Work out the finished part from the listing and answer in its coordinate system (mm). A direction names the side the tool comes from. Coordinates: 2 decimals unless noted, no trailing zeros. Write each loop counter-clockwise with the first axis right and the second up, starting at its lowest first coordinate (ties: lowest second). Pieces come first, ordered by that corner, then holes. Notation, with made-up numbers: (63.25, 73.25) - (112.25, 73.25) arc R9 ccw to (112.25, 83.25) - close; hole circle Ø1 at (74, -34). An arc over 180 degrees is marked (long way). Use a Markdown table: item, result. Add a question column.
(1) The part is cut by section A-A, the plane y = 5. Give the vertices of the cut face in (x, z), then the cut area to 3 significant figures.
(2) For a pull along Y with two mould halves and no side action, classify faces 4 (the face through (6, -1, 0)), 5 (the face through (20.74, 4.09, -0.64)), 6 (the face through (1.25, 5, 2.3)) as released by +Y, released by -Y, zero draft, split by the parting line, or undercut.
(3) Find the intervals of material crossed by line 1 (Y direction, x = 20.85, z = 0.55); line 2 (X direction, y = 0.75, z = 7.5); line 3 (X direction, y = 2.5, z = 1.75), in increasing order. Write a range as from..to.
(4) The part is cut by section B-B, the plane x = 3.5. Give the vertices of the cut face in (y, z).
(5) The part is cut by section C-C, the plane y = 0.75. Give the vertices of the cut face in (x, z).
(6) The part is cut by section D-D, the plane y = 7. Give the vertices of the cut face in (x, z), then the cut area to 3 significant figures.
(7) A tool of negligible diameter and unlimited length cuts with its end or side. For faces 1 (the face through (5.7, -0.5, 1.95)), 2 (the face through (20.25, 4, 2)), 3 (the face through (-1.948, -2.465, -0.086)), from which of +Z, -Z, +X, -X, +Y, -Y can it reach the whole face along a straight path? Write none if from no direction.
(8) Given pin 1 Ø0.5 at (x, y) = (7, -0.5) entering from +Z; pin 2 Ø5 at (x, z) = (9.5, 6) entering from +Y; pin 3 Ø3 at (x, z) = (7, -0.5) entering from -Y; pin 4 Ø4 at (x, z) = (13.5, 3.5) entering from -Y, each flat-ended and moving along its own axis, determine where each tip first touches the part or whether it passes through.
from build123d import *

# Parameters (mm, degrees)
SKETCH1_R             = 1.95
BOSS_EXTRUDE2_DEPTH   = 5
BOSS_EXTRUDE2_2_DEPTH = 5
SKETCH2_W             = 31
SKETCH2_H             = 15.95
BOSS_EXTRUDE4_DEPTH   = 2
CUT_EXTRUDE1_DEPTH    = 2
FILLET1_R             = 6
BOSS_EXTRUDE5_DEPTH   = 1
SKETCH6_W             = 1
SKETCH6_H             = 5
SKETCH6_W_2           = 5
BOSS_EXTRUDE6_DEPTH   = 6
SKETCH8_R             = 1.5
CUT_EXTRUDE3_DEPTH    = 26
FILLET5_R             = 1.5


with BuildPart() as part:
    # Sketch1 → Boss-Extrude2 (new body)
    with BuildSketch(Plane(origin=(0, 0, 0), x_dir=(1, 0, 0), z_dir=(0, 1, 0))):
        Circle(SKETCH1_R)
    extrude(amount=-BOSS_EXTRUDE2_DEPTH)



with BuildPart() as body_2:
    # Sketch1 → Boss-Extrude2 2 (new body)
    with BuildSketch(Plane(origin=(0, 0, 0), x_dir=(1, 0, 0), z_dir=(0, 1, 0))):
        with Locations((11.5, 0)):
            Circle(SKETCH1_R)
    extrude(amount=-BOSS_EXTRUDE2_2_DEPTH)


with BuildPart() as part_1:
    add(part.part)

    add(body_2.part)  # Boss-Extrude4 merges body 2
    # Sketch2 → Boss-Extrude4 (add)
    with BuildSketch(Plane(origin=(0, 0, 0), x_dir=(1, 0, 0), z_dir=(0, 1, 0))):
        with Locations((5.75, -6.025)):
            Rectangle(SKETCH2_W, SKETCH2_H)
    extrude(amount=BOSS_EXTRUDE4_DEPTH)

    # Sketch3 → Cut-Extrude1 (cut)
    with BuildSketch(Plane.XZ):
        with BuildLine():
            Line((0, 12.85), (15, 12.85))
            ThreePointArc((15, 12.85), (19.9, 7.95), (15, 3.05))
            Line((15, 3.05), (0, 3.05))
            ThreePointArc((0, 3.05), (-4.9, 7.95), (0, 12.85))
        make_face()
    extrude(amount=-CUT_EXTRUDE1_DEPTH, mode=Mode.SUBTRACT)

    # Fillet1
    fillet1_edges = [part_1.edges().sort_by_distance(p)[0] for p in [
        (-9.75, 1, 14),
        (21.25, 1, 14),
    ]]
    fillet(fillet1_edges, radius=FILLET1_R)

    # Sketch4 → Boss-Extrude5 (add)
    with BuildSketch(Plane.XZ):
        with BuildLine():
            Line((0, 1.95), (11.5, 1.95))
            ThreePointArc((11.5, 1.95), (13.45, 0), (11.5, -1.95))
            Line((11.5, -1.95), (0, -1.95))
            ThreePointArc((0, -1.95), (-1.95, 0), (0, 1.95))
        make_face()
    extrude(amount=BOSS_EXTRUDE5_DEPTH)

    # Sketch6 → Boss-Extrude6 (add)
    with BuildSketch(Plane(origin=(0, 2, 0), x_dir=(1, 0, 0), z_dir=(0, 1, 0))):
        with Locations((20.75, -0.55)):
            Rectangle(SKETCH6_W, SKETCH6_H)
        with Locations((-1.25, -0.55)):
            Rectangle(SKETCH6_W_2, SKETCH6_H)
    extrude(amount=BOSS_EXTRUDE6_DEPTH)

    # Sketch8 → Cut-Extrude3 (cut, through all)
    with BuildSketch(Plane.ZY.offset(3.75)):
        with Locations((0.55, 5)):
            Circle(SKETCH8_R)
    extrude(amount=-CUT_EXTRUDE3_DEPTH, mode=Mode.SUBTRACT)

    # Fillet5
    fillet5_edges = [part_1.edges().sort_by_distance(p)[0] for p in [
        (-1.875, 2, 3.05),
        (20.75, 2, 3.05),
    ]]
    fillet(fillet5_edges, radius=FILLET5_R)


solid = part_1.part
Model answer:
| question | item | result |
|---|---|---|
| 1 | outline | (-3.75, -1.95) - (1.25, -1.95) - (1.25, -0.95) - (-3.75, -0.95) - close; (-3.75, 2.05) - (1.25, 2.05) - (1.25, 3.05) - (-3.75, 3.05) - close; (20.25, -1.95) - (21.25, -1.95) - (21.25, -0.95) - (20.25, -0.95) - close; (20.25, 2.05) - (21.25, 2.05) - (21.25, 3.05) - (20.25, 3.05) - close |
| 1 | area | 12.0 mm^2 |
| 2 | face 4 | released by -Y |
| 2 | face 5 | undercut |
| 2 | face 6 | zero draft |
| 3 | line 1 | 0..3.5, 6.5..8 |
| 3 | line 2 | -9.75..-4.88, 19.88..21.25 |
| 3 | line 3 | -3.75..1.25, 20.25..21.25 |
| 4 | outline | (-1, -1.95) - (2, -1.95) - (2, 3.05) - (0, 3.05) - (0, 1.95) - (-1, 1.95) - close; (0, 12.85) - (2, 12.85) - (2, 14) - (0, 14) - close |
| 5 | outline | (-9.75, -1.95) - (21.25, -1.95) - (21.25, 8) arc R6 ccw to (15.25, 14) - (-3.75, 14) arc R6 ccw to (-9.75, 8) - close; hole (0, 3.05) - (15, 3.05) arc R4.9 ccw to (15, 12.85) - (0, 12.85) arc R4.9 ccw to start |
| 6 | outline | (-3.75, -1.95) - (1.25, -1.95) - (1.25, 3.05) - (-3.75, 3.05) - close; (20.25, -1.95) - (21.25, -1.95) - (21.25, 3.05) - (20.25, 3.05) - close |
| 6 | area | 30.0 mm^2 |
| 7 | face 1 | +Z, +X, -X, -Y |
| 7 | face 2 | +Z, -Z, +Y |
| 7 | face 3 | -Y |
| 8 | pin 1 | z = 1.95 |
| 8 | pin 2 | through |
| 8 | pin 3 | y = -1 |
| 8 | pin 4 | y = 0 |
